Source: CAD feature listing. Evaluate the final solid. Frame: model axes, mm. Face numbers are marked on the shaded views. A direction names the side the tool comes from. Round coordinates to 2 decimals unless told otherwise and drop trailing zeros. Order: outer loops, then holes, each group sorted by start corner. A loop starts at its lowest first (then second) coordinate and runs counter-clockwise, first axis right, second up. Notation, with made-up numbers: (41, 80.5) -> (83, 80.5) arc R22 cw to (83, 115.5) -> close; hole circle Ø3 at (74.5, 66.25). An arc over 180 degrees is marked (long way). One line per item, written item: value. Start each with the question number.
1) Pin query (flat end, axial travel): P1, Ø5.5, axis at x = 0, z = 0, coming from the +Y side; P2, Ø3, axis at y = 2.5, z = -23, coming from the +X side; P3, Ø3, axis at x = -1.5, z = -26.5, coming from the +Y side; P4, Ø4.5, axis at x = -0.5, z = -7, coming from the +Y side. Return the tip coordinate at first contact, or that it passes through.
2) Section A-A (x = 0). Return the cut outline in (y, z), and give its area (3 significant figures).
3) Section C-C (z = -0.5). Return the cut outline in (x, y).
4) Mould query, pull axis Z, two halves, no side actions, for the marked faces 6, 7 and 8. Classes: pulls with the +Z half, pulls with the -Z half, needs draft (parallel to the pull), parting line crosses it, or undercut.
5) Section B-B (y = 0.45). Return the cut outline in (x, z), and give its area (3 significant figures).
6) Ray query, L1, parallel to Z at x = 0, y = 1.75; L2, parallel to X at y = 1.8, z = 0; L3, parallel to X at y = 1.6, z = -25.65. Return the intervals inside material, ascending.
7) Section D-D (z = -12). Return the cut outline in (x, y).
8) Reachability of the marked faces 1, 2, 3, 4 and 5 from +Z, -Z, +X, -X, +Y, -Y: full face, straight path, thin tool, end or side. Return the list, or none.
Autodesk Inventor part; units mm, degrees
ref_plane "YZ Plane" through (0, 0, 0) normal (1, 0, 0) x (0, 1, 0)
ref_plane "XZ Plane" through (0, 0, 0) normal (0, 1, 0) x (-1, 0, 0)
ref_plane "XY Plane" through (0, 0, 0) normal (0, 0, 1) x (1, 0, 0)
sketch "Skizze1" plane through (0, 0, 0) normal (0, 1, 0) x (-1, 0, 0)
  circle A0 centre (0, 0) radius 4.45
  arc A1 (6.5, 0) -> (-6.5, 0) centre (0, 0) ccw
  line L0 (0, 0) -> (0, -17)
  line L1 (4, -14) -> (23.7753, -14) construction
  line L2 (0, 0) -> (0, -19.75)
  line L3 (0, 0) -> (0, -26.15)
  line L4 (0, 0) -> (0, -29.15)
  arc A2 (-3.2, -29.15) -> (3.2, -29.15) centre (0, -29.15) ccw
  line L5 (-3.2, -29.15) -> (-3.2, -24.95)
  line L6 (3.2, -29.15) -> (3.2, -26.15)
  line L7 (3.2, -26.15) -> (3.2, -17)
  line L8 (-3.2, -24.95) -> (-3.2, -23.5465)
  line L9 (-3.2, -23.5465) -> (-3.2, -17)
  line L10 (-3.2, -17) -> (-6.5, 0)
  line L11 (6.5, 0) -> (3.2, -17)
  line L12 (0, -29.15) -> (0, -25.65)
  arc A3 (-3.2, -25.65) -> (3.2, -25.65) centre (0, -25.65) ccw
  point P0 (3.2, -25.65)
  dimension "d0" = 8.9
  dimension "d1" = 13
  dimension "d2" = 17
  dimension "d27" = 6.4
  dimension "d35" = 3.5
extrude "Extrusion1" add sketch "Skizze1" along normal blind 3 contours A3 L5 L8 L9 L10 A1 L11 L7
sketch "Skizze2" plane through (0, 3, 0) normal (0, 1, 0) x (1, 0, 0)
  arc A0 (-6.5, 0) -> (6.5, 0) centre (0, 0) ccw
  line L0 (-3.2, 17) -> (-3.2, 19.75)
  line L1 (3.2, 17) -> (3.2, 19.75)
  line L2 (3.2, 26.15) -> (3.2, 19.75)
  line L3 (-3.2, 26.15) -> (-3.2, 19.75)
  arc A1 (3.2, 29.15) -> (-3.2, 29.15) centre (0, 29.15) ccw
  line L4 (3.2, 26.15) -> (3.2, 29.15)
  line L5 (-3.2, 26.15) -> (-3.2, 29.15)
  arc A2 (-6.5, 0) -> (6.5, 0) centre (0, 0) ccw
  line L6 (-3.2, 29.15) -> (-3.2, 17)
  line L7 (-6.5, 0) -> (-3.2, 17)
  line L8 (6.5, 0) -> (3.2, 17)
  line L9 (6.5, 0) -> (3.2, 17)
  circle A3 centre (0, 0) radius 4.45
  circle A4 centre (0, 0) radius 4.45
  line L10 (0, -4.45) -> (0, 14.55)
  arc A5 (2.482, 14.8497) -> (-2.482, 14.8497) centre (0, 14.55) ccw
  line L11 (-4.45, 0) -> (-2.4744, 14.9071)
  line L12 (4.45, 0) -> (2.4744, 14.9071)
  line L13 (-4.45, 0) -> (4.45, 0)
  line L14 (-4.45, 0) -> (-3.746, -5.312)
  line L15 (4.45, 0) -> (3.746, -5.312)
  arc A6 (3.2, 29.15) -> (-3.2, 29.15) centre (0, 29.15) ccw
  arc A7 (3.2, 25.65) -> (-3.2, 25.65) centre (0, 25.65) ccw
  arc A8 (3.2, 25.65) -> (-3.2, 25.65) centre (0, 25.65) ccw
  point P0 (-4.0763, 3.9842)
  point P1 (-5.7, 0)
  point P2 (0, 19.75)
  point P3 (-3.2, 26.15)
  point P4 (-2.4744, -14.9071)
  point P5 (2.4744, -14.9071)
  point P6 (-4.2964, -1.1592)
  point P7 (-4.2964, 1.1592)
  point P8 (4.2964, 1.1592)
  point P9 (4.2964, -1.1592)
  point P10 (3.2, 17)
  point P11 (-3.2, 26.65)
  point P12 (3.2, 26.65)
  dimension "d30" = 19
  dimension "d31" = 5
extrude "Extrusion2" add sketch "Skizze2" along normal blind 2.5 contours L7 L0 L3 A7 L2 L1 L8 A0 L15 A3 L12 A5 L11 L14
sketch "Skizze5" plane through (0, 0, 0) normal (0, -1, 0) x (1, 0, 0)
  line L0 (0, 0) -> (0, -29.15)
  circle A0 centre (0, -29.15) radius 1.5
  arc A1 (-3.2, -25.65) -> (3.2, -25.65) centre (0, -25.65) ccw
  line L1 (0, -29.15) -> (0, -25.65)
  circle A2 centre (0, -25.65) radius 1.5
  point P0 (-3.2, -26.65)
  dimension "d20" = 29.15
  dimension "d21" = 3
  dimension "d40" = 3.5
  dimension "d41" = 3
extrude "Extrusion5" cut sketch "Skizze5" against normal blind 6 contours A2 L0 | L0 A2
sketch "Skizze6" plane through (0, 5.5, 0) normal (0, 1, 0) x (1, 0, 0)
  arc A0 (3.2, 29.15) -> (-3.2, 29.15) centre (0, 29.15) ccw
  line L0 (-3.2, 29.15) -> (-3.2, 14)
  line L1 (-3.2, 29.15) -> (-3.2, 25.9472)
  arc A1 (3.2, 29.15) -> (-3.2, 29.15) centre (0, 29.15) ccw
  line L2 (3.2, 29.15) -> (3.2, 25.9472)
  line L3 (-3.2, 25.9472) -> (-3.2, 23.4472)
  line L4 (-3.2, 25.65) -> (-3.2, 17)
  line L5 (3.2, 17) -> (3.2, 25.65)
  arc A2 (3.2, 25.65) -> (-3.2, 25.65) centre (0, 25.65) ccw
  arc A3 (3.2, 26.65) -> (-3.2, 26.65) centre (0, 26.65) ccw
  line L6 (3.2, 17) -> (3.2, 25.65)
  line L7 (3.2, 26.65) -> (3.2, 23.4472)
  line L8 (-3.2, 23.4472) -> (-3.2, 22.4472)
  line L9 (-3.2, 25.65) -> (-3.2, 17)
  line L10 (-3.2, 22.4472) -> (3.2, 22.4472)
  line L11 (3.2, 23.4472) -> (3.2, 22.4472)
  point P0 (0, 0)
  dimension "d38" = 2.5
  dimension "d43" = 1
extrude "Extrusion6" cut sketch "Skizze6" against normal blind 1
sketch "Skizze7" plane through (0, 0, 0) normal (0, -1, 0) x (1, 0, 0)
  circle A0 centre (0, 0) radius 4.45
  line L0 (-6.6957, 4.45) -> (-6.6957, 6.6948)
  line L1 (-6.6957, 6.6948) -> (6.8805, 6.6948)
  line L2 (6.8805, 6.6948) -> (6.8805, 4.45)
  line L3 (6.8805, 4.45) -> (6.8805, 4.95)
  line L4 (6.8805, 4.95) -> (-6.6957, 4.95)
  dimension "d34" = 0.5
extrude "Extrusion7" cut sketch "Skizze7" against normal blind 20 contours L0 L1 L2 L4
properties part number "Servo_Exzenter_Smart_Neu_2"
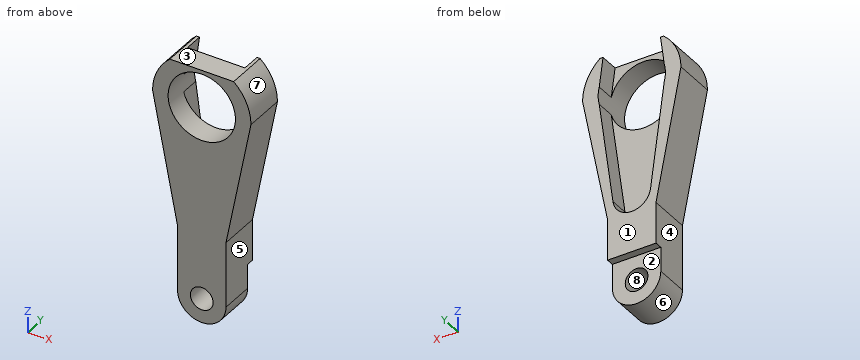
Findings:
1. P1: through
1. P2: x = 3.2
1. P3: y = 4.5
1. P4: y = 3
2. outline: (0, -28.85) -> (4.5, -28.85) -> (4.5, -27.15) -> (0, -27.15) -> close; (0, -24.15) -> (4.5, -24.15) -> (4.5, -22.45) -> (5.5, -22.45) -> (5.5, -17.05) -> (3, -17.05) -> (3, -4.45) -> (0, -4.45) -> close; (0, 4.45) -> (3, 4.45) -> (3, 4.95) -> (0, 4.95) -> close
2. area: 84.3 mm2
3. outline: (-6.4, 0) -> (-4.42, 0) -> (-4.42, 5.5) -> (-6.4, 5.5) -> close; (4.42, 0) -> (6.4, 0) -> (6.4, 5.5) -> (4.42, 5.5) -> close
4. face 6: pulls with the -Z half
4. face 7: pulls with the +Z half
4. face 8: undercut
5. outline: (-6.5, 0) -> (-3.2, -17) -> (-3.2, -25.65) arc R3.2 ccw to (3.2, -25.65) -> (3.2, -17) -> (6.5, 0) arc R6.5 ccw to (4.21, 4.95) -> (-4.21, 4.95) arc R6.5 ccw to start; hole circle Ø8.9 at (0, 0); hole circle Ø3 at (0, -25.65)
5. area: 224 mm2
6. L1: -28.85 to -27.15, -24.15 to -4.45, 4.45 to 4.95
6. L2: -6.5 to -4.45, 4.45 to 6.5
6. L3: -3.2 to -1.5, 1.5 to 3.2
7. outline: (-4.17, 0) -> (4.17, 0) -> (4.17, 5.5) -> (2.86, 5.5) -> (2.86, 3) -> (-2.86, 3) -> (-2.86, 5.5) -> (-4.17, 5.5) -> close
8. face 1: +Z, -Z, +X, -X, +Y
8. face 2: -Z, +X, -X, +Y
8. face 3: +Z, +X, -X, +Y, -Y
8. face 4: -Z, -X, +Y, -Y
8. face 5: -Z, +X, +Y, -Y
